Verification items for this drawing (mm, ordinates from the low corner). A direction names the side the tool comes from. Coordinates: 2 decimals unless noted, no trailing zeros. Loops run counter-clockwise (first coordinate to the right, second up) from the corner with the lowest first, then second, coordinate; pieces in that order, holes last. Notation, with made-up numbers: M -13,5.25 L 37,5.25 A14 ccw 37,20.25 Z; hole C 10.25,24 d7. An arc over 180 degrees is marked long. Use CSV: the item, a comma, the result in double quotes.
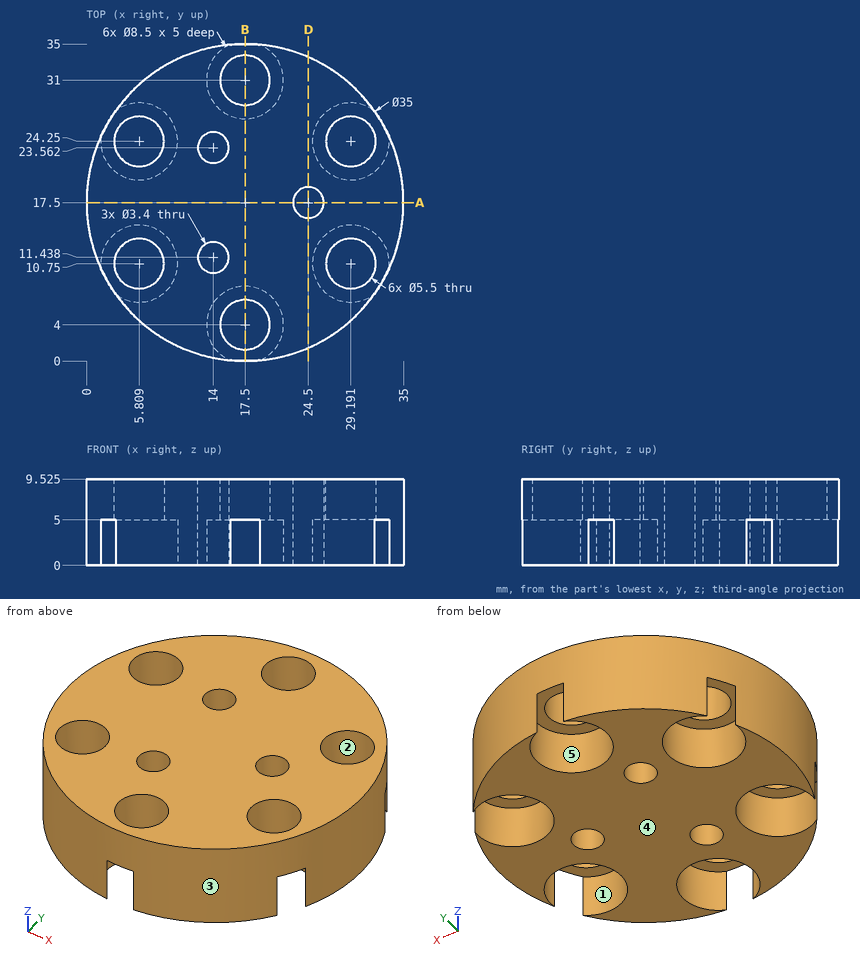
1. Section check A-A, the plane y = 17.5. Record the cut outline in (x, z) (1 decimal).
The answers:
outline,"M 0,0 L 22.8,0 L 22.8,9.5 L 0,9.5 Z; M 26.2,0 L 35,0 L 35,9.5 L 26.2,9.5 Z"
2. Set-up check for the marked faces 1 and 2: record each of +Z, -Z, +X, -X, +Y, -Y from which the full face is reachable in a straight line by a thin tool's end or side.
The answers:
face 1,"-Z"
face 2,"+Z, -Z"
3. Thickness scan on line 1 (Y direction, x = 17.5, z = 6.8); line 2 (X direction, y = 10.5, z = 6.25); line 3 (Y direction, x = 15, z = 8.5) (1 decimal). Record the ranges inside material, lowest first. Write a range as [from, to].
The answers:
line 1,"[0, 1.25], [6.75, 28.25], [33.75, 35]"
line 2,"[1.46, 3.07], [8.55, 12.58], [15.42, 26.45], [31.93, 33.54]"
line 3,"[0.2, 2.9], [5.1, 10.1], [12.8, 22.2], [24.9, 29.9], [32.1, 34.8]"
4. Gauge pin test, flat ends, axial feed: P1, Ø3, axis at x = 24.5, y = 17.5, coming from the +Z side; P2, Ø2, axis at y = 10.5, z = 7, coming from the -X side; P3, Ø2.5, axis at x = 19.5, y = 29, coming from the -Z side; P4, Ø3, axis at y = 7.5, z = 7.5, coming from the -X side. Record the tip position at first contact, or that the pin passes through.
The answers:
P1,"through"
P2,"x = 1.06"
P3,"z = 5"
P4,"x = 2.2"
5. Section check D-D, the plane x = 24.5. Record the cut outline in (y, z) (1 decimal).
The answers:
outline,"M 1.5,0 L 15.8,0 L 15.8,9.5 L 1.5,9.5 Z; M 19.2,0 L 33.5,0 L 33.5,9.5 L 19.2,9.5 Z"
6. Section check B-B, the plane x = 17.5. Count the separate pieces of the cut face and the enclosed holes in it, plus the area to 3 significant figures.
The answers:
separate pieces,"3"
enclosed holes,"0"
area,"201 mm^2"
7. Release check for a two-part mould opening along Y. For the marked faces 3, 4 and 5 record: +Y half, -Y half, draft (parallel to the pull), parting line (faces both ways), or undercut.
The answers:
face 3,"parting line"
face 4,"draft"
face 5,"undercut"
